Build history of the part. All positions in model axes, mm. Give positions to 0.01 mm unless a question says otherwise; leave off trailing zeros. Loops run counter-clockwise (first coordinate to the right, second up) from the corner with the lowest first, then second, coordinate; pieces in that order, holes last. Notation, with made-up numbers: M -27,-14.5 L 6,-14.5 A27 cw 6,17.5 Z; hole C 86,5.25 d2. An arc over 180 degrees is marked long. Answer as a JSON object with one key per item and string values. Group by question number.
1. Slice it at D-D (z = 15.5). List the corners of the cut face in (x, y), then the cut area to 3 significant figures.
2. Slice it at A-A (x = 55.5). List the corners of the cut face in (y, z).
3. Slice it at B-B (z = 26.5). List the corners of the cut face in (x, y), then the cut area to 3 significant figures.
4. Drop flat-ended pins along their axis: pin 1 Ø4 at (x, z) = (82.61, -6.6) entering from -Y; pin 2 Ø2 at (x, y) = (42.5, -0.5) entering from +Z. Give the stop position or say it passes through.
5. Slice it at C-C (y = -0.45). Give the number of separate pieces and of enclosed holes in the cut face, then the cut area to 3 significant figures.
6. Mould opens along Z. For faces 1 (the face through (87.144, 0.031, 2.532)), 2 (the face through (85.7, 0, -7.6)), 3 (the face through (96.683, 0.031, -25.544)), 4 (the face through (76.59, -0.03, -38.32)) say: released by +Z, released by -Z, zero draft, split by the parting line, or undercut.
7. Drill centre lines: line 1 along Z through (x, y) = (72, 0.85); line 2 along X through (y, z) = (-1.75, -16); line 3 along X through (y, z) = (-0.95, -16.5). Where is each one in solid material? Low to high. Write a range as [from, to].
from build123d import *

# Parameters (mm, degrees)
BOSS_EXTRUDE1_DEPTH             = 2.25
BOSS_EXTRUDE2_DEPTH             = 2.25
BOSS_EXTRUDE3_DEPTH             = 2.25
CUT_EXTRUDE1_START              = -5.5
SKETCH2_R                       = 2.25
CUT_EXTRUDE1_DEPTH              = 6.5
CIRPATTERN1_COUNT               = 3
CIRPATTERN1_ANGLE               = 60
CIRPATTERN1_THE_OTHER_WAY_COUNT = 3
CIRPATTERN1_THE_OTHER_WAY_ANGLE = 60
CUT_EXTRUDE2_START              = -5.5
SKETCH6_R                       = 3.25
CUT_EXTRUDE2_DEPTH              = 6.5
LPATTERN1_COUNT                 = 3
LPATTERN1_PITCH                 = 12.5
SKETCH7_R                       = 3.25
CUT_EXTRUDE3_DEPTH              = 10
LPATTERN2_COUNT                 = 4
LPATTERN2_PITCH                 = 12


with BuildPart() as part:
    # Sketch1 → Boss-Extrude1 (new body, symmetric)
    with BuildSketch(Plane(origin=(0, 0, 0), x_dir=(1, 0, 0), z_dir=(0, 1, 0))):
        with BuildLine():
            Line((0, 33), (0, 43))
            ThreePointArc((0, 43), (41.53481053, 11.129218939), (21.5, -37.239092363))
            Line((21.5, -37.239092363), (16.5, -28.578838325))
            ThreePointArc((16.5, -28.578838325), (31.875552268, 8.541028488), (0, 33))
        make_face()
    extrude(amount=BOSS_EXTRUDE1_DEPTH, both=True)

    # Sketch4 → Boss-Extrude2 (add, symmetric)
    with BuildSketch(Plane(origin=(0, 0, 0), x_dir=(1, 0, 0), z_dir=(0, 1, 0))):
        Polygon((90.122106501, 50.030050167), (25.40507614, 32.689174146), (38.346028395, -15.607117169), (103.063058756, 1.733758853), align=None)
    extrude(amount=BOSS_EXTRUDE2_DEPTH, both=True)

    # Sketch5 → Boss-Extrude3 (add, symmetric)
    with BuildSketch(Plane(origin=(0, 0, 0), x_dir=(1, 0, 0), z_dir=(0, 1, 0))):
        Polygon((0, 43), (58.722616268, 41.616582117), (27.323126035, 33.203114066), align=None)
        Polygon((71.663568523, -6.679709198), (40.26407829, -15.093177248), (21.5, -37.239092363), align=None)
    extrude(amount=BOSS_EXTRUDE3_DEPTH, both=True)

    # Sketch2 → Cut-Extrude1 (cut)
    with BuildSketch(Plane(origin=(0, 2.25, 0), x_dir=(1, 0, 0), z_dir=(0, 1, 0)).offset(CUT_EXTRUDE1_START)):
        with Locations((36.757261811, 9.638656763)):
            Circle(SKETCH2_R)
    cut_extrude1 = extrude(amount=CUT_EXTRUDE1_DEPTH, mode=Mode.SUBTRACT)

    # CirPattern1: Cut-Extrude1 ×3 about axis
    cirpattern1_axis = Axis((0, 0, 0), (0, -1, 0))
    for i in range(1, CIRPATTERN1_COUNT):
        add(cut_extrude1.rotate(cirpattern1_axis, i * CIRPATTERN1_ANGLE / (CIRPATTERN1_COUNT - 1)), mode=Mode.SUBTRACT)

    # CirPattern1 the other way: Cut-Extrude1 ×3 about axis
    cirpattern1_the_other_way_axis = Axis((0, 0, 0), (0, 1, 0))
    for i in range(1, CIRPATTERN1_THE_OTHER_WAY_COUNT):
        add(cut_extrude1.rotate(cirpattern1_the_other_way_axis, i * CIRPATTERN1_THE_OTHER_WAY_ANGLE / (CIRPATTERN1_THE_OTHER_WAY_COUNT - 1)), mode=Mode.SUBTRACT)

    # Sketch6 → Cut-Extrude2 (cut)
    with BuildSketch(Plane(origin=(0, 2.25, 0), x_dir=(1, 0, 0), z_dir=(0, 1, 0)).offset(CUT_EXTRUDE2_START)):
        with Locations((94.679313348, 9.840102845)):
            Circle(SKETCH6_R)
        with Locations((86.914741995, 38.817877634)):
            Circle(SKETCH6_R)
    cut_extrude2 = extrude(amount=CUT_EXTRUDE2_DEPTH, mode=Mode.SUBTRACT)

    # LPattern1: Cut-Extrude2 ×3
    with Locations(*[Vector(-0.965925826, 0, 0.258819045) * (i * LPATTERN1_PITCH) for i in range(1, LPATTERN1_COUNT)]):
        add(cut_extrude2, mode=Mode.SUBTRACT)

    # Sketch7 → Cut-Extrude3 (cut)
    with BuildSketch(Plane(origin=(0, 2.25, 0), x_dir=(1, 0, 0), z_dir=(0, 1, 0))):
        with Locations((90.797027671, 24.32899024)):
            Circle(SKETCH7_R)
    cut_extrude3 = extrude(amount=-CUT_EXTRUDE3_DEPTH, mode=Mode.SUBTRACT)

    # LPattern2: Cut-Extrude3 ×4
    with Locations(*[Vector(-0.965925826, 0, 0.258819045) * (i * LPATTERN2_PITCH) for i in range(1, LPATTERN2_COUNT)]):
        add(cut_extrude3, mode=Mode.SUBTRACT)


solid = part.part
Established:
{
 "1": {"outline": "M 29.13,-2.25 L 57.18,-2.25 L 57.18,2.25 L 29.13,2.25 Z", "area": "126 mm^2"},
 "2": {"outline": "M -2.25,-41.69 L 2.25,-41.69 L 2.25,-18.22 L -2.25,-18.22 Z; M -2.25,-11.8 L 2.25,-11.8 L 2.25,16.53 L -2.25,16.53 Z"},
 "3": {"outline": "M 19.67,-2.25 L 24.54,-2.25 L 24.54,2.25 L 19.67,2.25 Z; M 28.92,-2.25 L 39.13,-2.25 L 39.13,2.25 L 28.92,2.25 Z", "area": "67.9 mm^2"},
 "4": {"pin 1": "passes through", "pin 2": "stops at z = 25.06"},
 "5": {"separate pieces": "1", "enclosed holes": "15", "area": "4,000 mm^2"},
 "6": {"face 1": "released by +Z", "face 2": "undercut", "face 3": "released by -Z", "face 4": "undercut"},
 "7": {"line 1": "z = [-45.17, -37.16], [-34, -6.27], [-0.47, 6.59]", "line 2": "x = [28.86, 52.93], [59.12, 65.15], [70.08, 99.24]", "line 3": "x = [28.58, 53.13], [58.91, 64.8], [70.43, 99.11]"}
}
